Geometry check sheet. Reference: the model listing, model coordinates, mm. Face numbers are marked on the shaded views. A direction names the side the tool comes from. Give positions to 0.01 mm unless a question says otherwise; leave off trailing zeros. Write each loop counter-clockwise with the first axis right and the second up, starting at its lowest first coordinate (ties: lowest second). Pieces come first, ordered by that corner, then holes.
(1) Cross-section at B-B (x = 75.75). Record the boundary of the cut face in (y, z).
(2) Tool access check on the marked faces 1, 2 and 3. Record the directions out of +Z, -Z, +X, -X, +Y, -Y that give a thin tool (end or side, any length) a straight path to the whole face; none if there is none.
(3) Thickness scan on line 1 along Y through (x, z) = (68.25, 52.5); line 2 along Z through (x, y) = (57.5, 34); line 3 along Z through (x, y) = (67, 42.5). Record the ranges inside material, lowest first.
(4) Cross-section at A-A (z = 47.5). Record the boundary of the cut face in (x, y), and give its area (3 significant figures).
(5) Cross-section at C-C (y = 11.5). Record the boundary of the cut face in (x, z).
(6) Depth check by flat-ended pin: P1, Ø1.9, axis at x = 71.24, y = -44.51, coming from the +Z side; P2, Ø3, axis at x = 57, y = 26.5, coming from the -Z side; P3, Ø3.5, axis at x = 67.09, y = -50.55, coming from the +Z side; P4, Ø2, axis at x = 58.5, z = 8.5, coming from the -Y side. Enter the tip coordinate at first touch or a pass-through.
(7) Mould release check, pull along Y, two halves, no side actions. Record for the marked faces 4, 5 and 6: +Y half, -Y half, draft (parallel to the pull), parting line (faces both ways), or undercut.
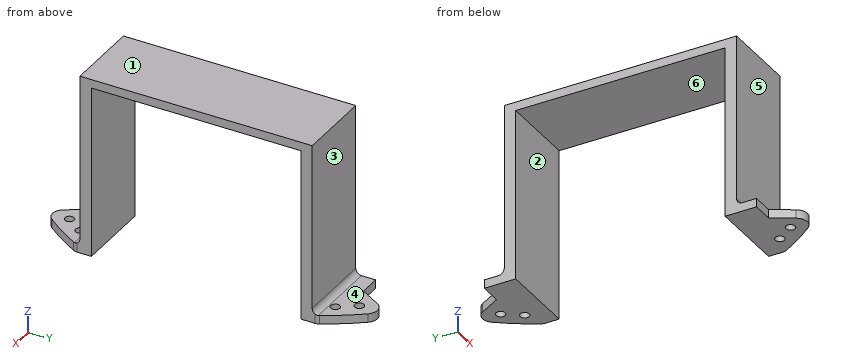
```python
from build123d import *

# Parameters (mm, degrees)
BOSS_EXTRUDE1_OUTLINE_R = 1.6
BOSS_EXTRUDE1_DEPTH     = 3
SKETCH4_W               = 26.662281873
SKETCH4_H               = 4
BOSS_EXTRUDE2_DEPTH     = 57
SKETCH5_W               = 26.662281873
SKETCH5_H               = 81.026436392
BOSS_EXTRUDE3_DEPTH     = 3
FILLET3_R               = 2


# Read off the part's stored shape, not the designer's step: Boss-Extrude1
with BuildPart() as part:
    # Boss-Extrude1 outline → Boss-Extrude1 (new body)
    # profile 1 of 2: a face of its own
    with BuildSketch(Plane.XY):
        with BuildLine():
            ThreePointArc((63.289582375, -54.620772264), (66.466019523, -56.610414999), (69.895033825, -55.0970439))
            ThreePointArc((69.895033825, -55.0970439), (74.189882191, -49.161584399), (77.981994569, -42.892989206))
            ThreePointArc((77.981994569, -42.892989206), (78.25905658, -42.193542837), (78.353388011, -41.447158109))
            Line((78.353388011, -41.447158109), (78.353388011, -36.513218196))
            Line((78.353388011, -36.513218196), (51.691106138, -36.513218196))
            Line((51.691106138, -36.513218196), (51.691106138, -47.469854476))
            Line((51.691106138, -47.469854476), (59.160998066, -47.469854476))
            Line((59.160998066, -47.469854476), (63.289582375, -54.620772264))
        make_face()
        with Locations((67.085382844, -50.552461945)):
            Circle(BOSS_EXTRUDE1_OUTLINE_R, mode=Mode.SUBTRACT)
        with Locations((71.236040077, -44.513218196)):
            Circle(BOSS_EXTRUDE1_OUTLINE_R, mode=Mode.SUBTRACT)
    # profile 2 of 2: a face of its own
    with BuildSketch(Plane.XY):
        with BuildLine():
            Line((78.353388011, 36.513218196), (78.353388011, 41.447158109))
            ThreePointArc((78.353388011, 41.447158109), (78.25905658, 42.193542837), (77.981994569, 42.892989206))
            ThreePointArc((77.981994569, 42.892989206), (74.189882191, 49.161584398), (69.895033826, 55.0970439))
            ThreePointArc((69.895033826, 55.0970439), (66.466019523, 56.610414999), (63.289582375, 54.620772264))
            Line((63.289582375, 54.620772264), (59.160998066, 47.469854476))
            Line((59.160998066, 47.469854476), (51.691106138, 47.469854476))
            Line((51.691106138, 47.469854476), (51.691106138, 36.513218196))
            Line((51.691106138, 36.513218196), (78.353388011, 36.513218196))
        make_face()
        with Locations((67.085382844, 50.552461945)):
            Circle(BOSS_EXTRUDE1_OUTLINE_R, mode=Mode.SUBTRACT)
        with Locations((71.236040077, 44.513218196)):
            Circle(BOSS_EXTRUDE1_OUTLINE_R, mode=Mode.SUBTRACT)
    extrude(amount=BOSS_EXTRUDE1_DEPTH)

    # Sketch4 → Boss-Extrude2 (add)
    with BuildSketch(Plane.XY.offset(3)):
        with Locations((65.022247075, 38.513218196)):
            Rectangle(SKETCH4_W, SKETCH4_H)
        with Locations((65.022247075, -38.513218196)):
            Rectangle(SKETCH4_W, SKETCH4_H)
    extrude(amount=BOSS_EXTRUDE2_DEPTH)

    # Sketch5 → Boss-Extrude3 (add)
    with BuildSketch(Plane.XY.offset(60)):
        with Locations((65.022247075, 0)):
            Rectangle(SKETCH5_W, SKETCH5_H)
    extrude(amount=BOSS_EXTRUDE3_DEPTH)

    # Fillet3
    fillet3_edges = [part.edges().sort_by_distance(p)[0] for p in [
        (65.022247075, -40.513218196, 3),
        (65.022247075, 40.513218196, 3),
    ]]
    fillet(fillet3_edges, radius=FILLET3_R)


solid = part.part
```
Reply:
1. outline: (-46.72, 0) - (-36.51, 0) - (-36.51, 60) - (36.51, 60) - (36.51, 0) - (46.72, 0) - (46.72, 3) - (42.51, 3) arc R2 cw to (40.51, 5) - (40.51, 63) - (-40.51, 63) - (-40.51, 5) arc R2 cw to (-42.51, 3) - (-46.72, 3) - close
2. face 1: +Z, +X, -X, +Y, -Y
2. face 2: -Z, +X, -X
2. face 3: +Z, +X, -X, +Y
3. line 1: y = -40.51 to -36.51, 36.51 to 40.51
3. line 2: z = 60 to 63
3. line 3: z = 0 to 3
4. outline: (51.69, -40.51) - (78.35, -40.51) - (78.35, -36.51) - (51.69, -36.51) - close; (51.69, 36.51) - (78.35, 36.51) - (78.35, 40.51) - (51.69, 40.51) - close
4. area: 213 mm2
5. outline: (51.69, 60) - (78.35, 60) - (78.35, 63) - (51.69, 63) - close
6. P1: passes through
6. P2: stops at z = 60
6. P3: stops at z = 3
6. P4: stops at y = -40.51
7. face 4: draft
7. face 5: -Y half
7. face 6: undercut
